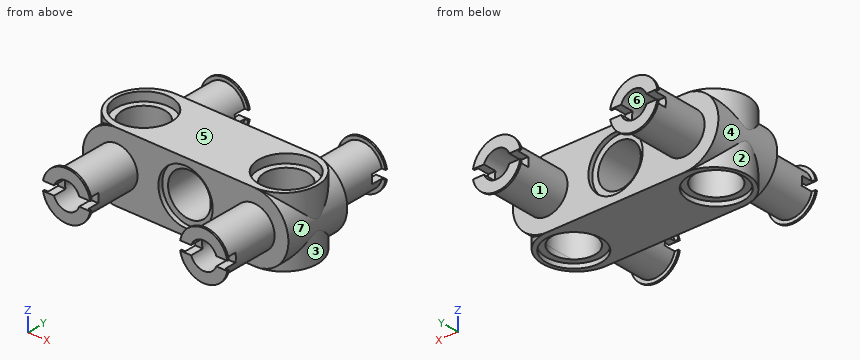
```python
from build123d import *

# Parameters (mm, degrees)
SKETCH2_R           = 2.4
BOSS_EXTRUDE1_DEPTH = 7.7
SKETCH4_R           = 2.4
CUT_EXTRUDE1_DEPTH  = 7.7
SKETCH7_R           = 3.05
SKETCH7_R_2         = 2.4
CUT_EXTRUDE2_DEPTH  = 0.5
SKETCH8_R           = 2.3
BOSS_EXTRUDE2_DEPTH = 6.5
SKETCH9_R           = 1.5
CUT_EXTRUDE3_DEPTH  = 6.5
BOSS_EXTRUDE4_START = -3.85
SKETCH10_R          = 3.05
BOSS_EXTRUDE4_DEPTH = 3.85
SKETCH13_R          = 2.7
SKETCH13_R_2        = 2.3
BOSS_EXTRUDE6_DEPTH = 0.2
CUT_EXTRUDE4_START  = -0.5
SKETCH14_R          = 3.1
SKETCH14_R_2        = 2.4
CUT_EXTRUDE4_DEPTH  = 0.5
SKETCH16_W          = 27.88395247
SKETCH16_H          = 1
CUT_EXTRUDE5_DEPTH  = 1.5
MIRROR5_OUTLINE_R   = 3.1
MIRROR5_DEPTH       = 0.5
MIRROR5_START       = 6.7
MIRROR5_2_OUTLINE_R = 3.1
MIRROR5_2_DEPTH     = 0.5
SKETCH17_R          = 2.4
CUT_EXTRUDE6_DEPTH  = 18.285326258


# Read off the part's stored shape, not the designer's step: Mirror5
with BuildPart() as part:
    # Sketch2 → Boss-Extrude1 (new body)
    with BuildSketch(Plane.XY):
        with BuildLine():
            Line((7.7, -3.8), (-7.7, -3.8))
            ThreePointArc((-7.7, -3.8), (-11.5, 0), (-7.7, 3.8))
            Line((-7.7, 3.8), (7.7, 3.8))
            ThreePointArc((7.7, 3.8), (11.5, 0), (7.7, -3.8))
        make_face()
        with Locations(Location((8, 0, 0), (0, 0, 180))):
            Circle(SKETCH2_R, mode=Mode.SUBTRACT)
        with Locations(Location((-8, 0, 0), (0, 0, 180))):
            Circle(SKETCH2_R, mode=Mode.SUBTRACT)
    extrude(amount=BOSS_EXTRUDE1_DEPTH)

    # Sketch4 → Cut-Extrude1 (cut)
    with BuildSketch(Plane(origin=(0, 3.8, 0), x_dir=(1, 0, 0), z_dir=(0, 1, 0))):
        with Locations(Location((0, -3.85, 0), (0, 0, 180))):
            Circle(SKETCH4_R)
    extrude(amount=-CUT_EXTRUDE1_DEPTH, mode=Mode.SUBTRACT)

    # Sketch7 → Cut-Extrude2 (cut)
    with BuildSketch(Plane(origin=(0, 3.8, 0), x_dir=(1, 0, 0), z_dir=(0, 1, 0))):
        with Locations(Location((0, -3.85, 0), (0, 0, 180))):
            Circle(SKETCH7_R)
        with Locations(Location((0, -3.85, 0), (0, 0, 180))):
            Circle(SKETCH7_R_2, mode=Mode.SUBTRACT)
    cut_extrude2 = extrude(amount=-CUT_EXTRUDE2_DEPTH, mode=Mode.SUBTRACT)

    # Mirror1: Cut-Extrude2 across plane
    add(cut_extrude2.mirror(Plane.ZX), mode=Mode.SUBTRACT)

    # Sketch8 → Boss-Extrude2 (add)
    with BuildSketch(Plane(origin=(0, 3.8, 0), x_dir=(1, 0, 0), z_dir=(0, 1, 0))):
        with Locations(Location((7.7, -3.85, 0), (0, 0, 270))):
            Circle(SKETCH8_R)
        with Locations((-7.7, -3.85)):
            Circle(SKETCH8_R)
    boss_extrude2 = extrude(amount=BOSS_EXTRUDE2_DEPTH)

    # Sketch9 → Cut-Extrude3 (cut)
    with BuildSketch(Plane(origin=(0, 10.3, 0), x_dir=(1, 0, 0), z_dir=(0, 1, 0))):
        with Locations(Location((7.7, -3.85, 0), (0, 0, 180))):
            Circle(SKETCH9_R)
        with Locations(Location((-7.7, -3.85, 0), (0, 0, 180))):
            Circle(SKETCH9_R)
    cut_extrude3 = extrude(amount=-CUT_EXTRUDE3_DEPTH, mode=Mode.SUBTRACT)

    # Sketch10 → Boss-Extrude4 (add)
    # profile 1 of 3: a face of its own
    with BuildSketch(Plane(origin=(0, 3.8, 0), x_dir=(1, 0, 0), z_dir=(0, 1, 0)).offset(BOSS_EXTRUDE4_START)):
        with BuildLine():
            ThreePointArc((-7.7, 0), (-11.55, -3.85), (-7.7, -7.7))
            Line((-7.7, -7.7), (-7.7, -6.15))
            ThreePointArc((-7.7, -6.15), (-5.4, -3.85), (-7.7, -1.55))
            Line((-7.7, -1.55), (-7.7, 0))
        make_face()
    # profile 2 of 3: a face of its own
    with BuildSketch(Plane(origin=(0, 3.8, 0), x_dir=(1, 0, 0), z_dir=(0, 1, 0)).offset(BOSS_EXTRUDE4_START)):
        with BuildLine():
            Line((7.7, -7.7), (7.7, -6.15))
            ThreePointArc((7.7, -6.15), (5.4, -3.85), (7.7, -1.55))
            Line((7.7, -1.55), (7.7, 0))
            Line((7.7, 0), (-7.7, 0))
            Line((-7.7, 0), (-7.7, -1.55))
            ThreePointArc((-7.7, -1.55), (-5.4, -3.85), (-7.7, -6.15))
            Line((-7.7, -6.15), (-7.7, -7.7))
            Line((-7.7, -7.7), (7.7, -7.7))
        make_face()
        with Locations(Location((0, -3.85, 0), (0, 0, 180))):
            Circle(SKETCH10_R, mode=Mode.SUBTRACT)
    # profile 3 of 3: a face of its own
    with BuildSketch(Plane(origin=(0, 3.8, 0), x_dir=(1, 0, 0), z_dir=(0, 1, 0)).offset(BOSS_EXTRUDE4_START)):
        with BuildLine():
            ThreePointArc((7.7, 0), (11.55, -3.85), (7.7, -7.7))
            Line((7.7, -7.7), (7.7, -6.15))
            ThreePointArc((7.7, -6.15), (5.4, -3.85), (7.7, -1.55))
            Line((7.7, -1.55), (7.7, 0))
        make_face()
    boss_extrude4 = extrude(amount=BOSS_EXTRUDE4_DEPTH)

    # Mirror2: Boss-Extrude2, Cut-Extrude3, Boss-Extrude4 across plane
    add(boss_extrude2.mirror(Plane.ZX))
    add(cut_extrude3.mirror(Plane.ZX), mode=Mode.SUBTRACT)
    add(boss_extrude4.mirror(Plane.ZX))

    # Sketch13 → Boss-Extrude6 (add)
    # profile 1 of 2: a face of its own
    with BuildSketch(Plane(origin=(0, 10.1, 0), x_dir=(1, 0, 0), z_dir=(0, 1, 0))):
        with Locations(Location((-7.7, -3.85, 0), (0, 0, 180))):
            Circle(SKETCH13_R)
        with Locations((-7.7, -3.85)):
            Circle(SKETCH13_R_2, mode=Mode.SUBTRACT)
    # profile 2 of 2: a face of its own
    with BuildSketch(Plane(origin=(0, 10.1, 0), x_dir=(1, 0, 0), z_dir=(0, 1, 0))):
        with Locations(Location((7.7, -3.85, 0), (0, 0, 180))):
            Circle(SKETCH13_R)
        with Locations((7.7, -3.85)):
            Circle(SKETCH13_R_2, mode=Mode.SUBTRACT)
    boss_extrude6 = extrude(amount=BOSS_EXTRUDE6_DEPTH)

    # Sketch14 → Cut-Extrude4 (cut)
    # profile 1 of 2: a face of its own
    with BuildSketch(Plane.XY.offset(7.7).offset(CUT_EXTRUDE4_START)):
        with Locations((-8, 0)):
            Circle(SKETCH14_R)
        with Locations((-8, 0)):
            Circle(SKETCH14_R_2, mode=Mode.SUBTRACT)
    # profile 2 of 2: a face of its own
    with BuildSketch(Plane.XY.offset(7.7).offset(CUT_EXTRUDE4_START)):
        with Locations(Location((8, 0, 0), (0, 0, 180))):
            Circle(SKETCH14_R)
        with Locations((8, 0)):
            Circle(SKETCH14_R_2, mode=Mode.SUBTRACT)
    extrude(amount=CUT_EXTRUDE4_DEPTH, mode=Mode.SUBTRACT)

    # Mirror3: Boss-Extrude6 across plane
    add(boss_extrude6.mirror(Plane.ZX))

    # Sketch16 → Cut-Extrude5 (cut)
    with BuildSketch(Plane(origin=(0, 10.3, 0), x_dir=(1, 0, 0), z_dir=(0, 1, 0))):
        with Locations((0, -3.85)):
            Rectangle(SKETCH16_W, SKETCH16_H)
    cut_extrude5 = extrude(amount=-CUT_EXTRUDE5_DEPTH, mode=Mode.SUBTRACT)

    # Mirror4: Cut-Extrude5 across plane
    add(cut_extrude5.mirror(Plane.ZX), mode=Mode.SUBTRACT)

    # Mirror5 outline → Mirror5 (cut)
    # profile 1 of 2: a face of its own
    with BuildSketch(Plane.XY):
        with Locations((-8, 0)):
            Circle(MIRROR5_OUTLINE_R)
        with BuildLine():
            ThreePointArc((-10.288436326, 0.723228306), (-5.6, 7.56e-07), (-10.28843587, -0.72322975))
            ThreePointArc((-10.28843587, -0.72322975), (-10.4, -7.57e-07), (-10.288436326, 0.723228306))
        make_face(mode=Mode.SUBTRACT)
    # profile 2 of 2: a face of its own
    with BuildSketch(Plane.XY):
        with Locations((8, 0)):
            Circle(MIRROR5_OUTLINE_R)
        with BuildLine():
            ThreePointArc((10.28843587, -0.72322975), (5.6, 7.56e-07), (10.288436326, 0.723228306))
            ThreePointArc((10.288436326, 0.723228306), (10.4, -7.57e-07), (10.28843587, -0.72322975))
        make_face(mode=Mode.SUBTRACT)
    extrude(amount=MIRROR5_DEPTH, mode=Mode.SUBTRACT)

    # Mirror5 2 outline → Mirror5 2 (cut)
    # profile 1 of 2: a face of its own
    with BuildSketch(Plane.XY.offset(MIRROR5_START)):
        with Locations((-8, 0)):
            Circle(MIRROR5_2_OUTLINE_R)
        with BuildLine():
            ThreePointArc((-10.288436326, 0.723228306), (-5.6, 7.56e-07), (-10.28843587, -0.72322975))
            ThreePointArc((-10.28843587, -0.72322975), (-10.4, -7.57e-07), (-10.288436326, 0.723228306))
        make_face(mode=Mode.SUBTRACT)
    # profile 2 of 2: a face of its own
    with BuildSketch(Plane.XY.offset(MIRROR5_START)):
        with Locations((8, 0)):
            Circle(MIRROR5_2_OUTLINE_R)
        with BuildLine():
            ThreePointArc((10.28843587, -0.72322975), (5.6, 7.56e-07), (10.288436326, 0.723228306))
            ThreePointArc((10.288436326, 0.723228306), (10.4, -7.57e-07), (10.28843587, -0.72322975))
        make_face(mode=Mode.SUBTRACT)
    extrude(amount=MIRROR5_2_DEPTH, mode=Mode.SUBTRACT)

    # Sketch17 → Cut-Extrude6 (cut, through all)
    with BuildSketch(Plane(origin=(0, 0, 0), x_dir=(-1, 0, 0), z_dir=(0, 0, -1))):
        with Locations((-8, 0)):
            Circle(SKETCH17_R)
        with Locations((8, 0)):
            Circle(SKETCH17_R)
    extrude(amount=-CUT_EXTRUDE6_DEPTH, mode=Mode.SUBTRACT)


solid = part.part
```
Input: part model. Units: mm. Frame: model coordinates. Face numbers are marked on the shaded views. A direction names the side the tool comes from. Round coordinates to 2 decimals unless told otherwise and drop trailing zeros. Write each loop counter-clockwise with the first axis right and the second up, starting at its lowest first coordinate (ties: lowest second). Pieces come first, ordered by that corner, then holes. Notation, with made-up numbers: (-30.75, -36.75) -> (-14.75, -36.75) arc R28 ccw to (-14.75, -3.75) -> close; hole circle Ø8 at (-25, -4.75). An arc over 180 degrees is marked (long way). Answer as CSV lines item,"result".
1. Ray query, L1, parallel to X at y = -5.5, z = 3.85; L2, parallel to Z at x = 7.7, y = -6.75; L3, parallel to Y at x = -8, z = 7.1. Return the intervals inside material, ascending. Write a range as [from, to].
Geometry says:
L1,"x = [-10, -9.2], [-6.2, -5.4], [5.4, 6.2], [9.2, 10]"
L2,"z = [1.55, 2.35], [5.35, 6.15]"
L3,"y = [-3.8, -3.1], [3.1, 3.8]"
2. Mould query, pull axis Z, two halves, no side actions, for the marked faces 5, 6 and 7. Classes: +Z half, -Z half, draft (parallel to the pull), parting line (faces both ways), or undercut.
Geometry says:
face 5,"+Z half"
face 6,"undercut"
face 7,"parting line"
3. Section A-A (x = 0). Return the cut outline in (y, z).
Geometry says:
outline,"(-3.8, 0) -> (3.8, 0) -> (3.8, 0.8) -> (3.3, 0.8) -> (3.3, 1.45) -> (-3.3, 1.45) -> (-3.3, 0.8) -> (-3.8, 0.8) -> close; (-3.8, 6.9) -> (-3.3, 6.9) -> (-3.3, 6.25) -> (3.3, 6.25) -> (3.3, 6.9) -> (3.8, 6.9) -> (3.8, 7.7) -> (-3.8, 7.7) -> close"
4. Reachability of the marked faces 1, 2, 3 and 4 from +Z, -Z, +X, -X, +Y, -Y: full face, straight path, thin tool, end or side. Return the list, or none.
Geometry says:
face 1,"none"
face 2,"-Z, -X"
face 3,"-Z, +X"
face 4,"-X"
5. Section C-C (z = 3.85). Give the number of separate pieces and of enclosed holes in the cut face, plus the area to 3 significant figures.
Geometry says:
separate pieces,"2"
enclosed holes,"2"
area,"134 mm^2"
6. Contact query for flat-ended pins moving along their axis: P1, Ø0.6, axis at x = -5.5, y = 9.5, coming from the +Z side; P2, Ø1, axis at x = -5.5, y = 9.5, coming from the -Z side; P3, Ø0.6, axis at x = 9.5, y = -9.5, coming from the +Z side. Output: stop coordinate, or through.
Geometry says:
P1,"stops at z = 5.15"
P2,"stops at z = 2.3"
P3,"stops at z = 5.59"
7. Section B-B (y = 5). Return the cut outline in (x, z), plus the area to 3 significant figures.
Geometry says:
outline,"circle Ø4.6 at (-7.7, 3.85); circle Ø4.6 at (7.7, 3.85); hole circle Ø3 at (-7.7, 3.85); hole circle Ø3 at (7.7, 3.85)"
area,"19.1 mm^2"
